Here's how the part is built. I have some questions about the finished solid (model axes, mm). Face numbers are marked on the shaded views. A direction names the side the tool comes from. Coordinates: 2 decimals unless noted, no trailing zeros. Write each loop counter-clockwise with the first axis right and the second up, starting at its lowest first coordinate (ties: lowest second). Pieces come first, ordered by that corner, then holes.
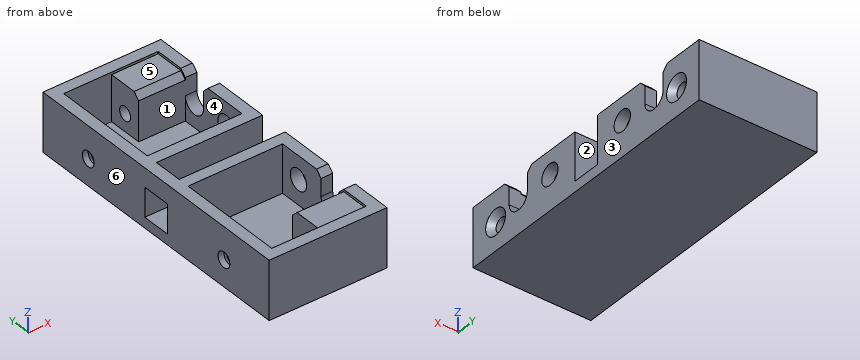
Autodesk Inventor part; units mm, degrees
ref_plane "YZ Plane" through (0, 0, 0) normal (1, 0, 0) x (0, 1, 0)
ref_plane "XZ Plane" through (0, 0, 0) normal (0, 1, 0) x (-1, 0, 0)
ref_plane "XY Plane" through (0, 0, 0) normal (0, 0, 1) x (1, 0, 0)
sketch "Sketch3" plane through (0, 0, 0) normal (0, 0, 1) x (1, 0, 0)
  line L0 (-10.1, 25) -> (10.1, 25)
  line L1 (10.1, 25) -> (10.1, -25)
  line L2 (10.1, -25) -> (-10.1, -25)
  line L3 (-10.1, -25) -> (-10.1, 25)
  point P0 (0, 0)
  dimension "d26" = 20.2
  dimension "d27" = 50
extrude "Extrusion3" add sketch "Sketch3" along normal blind 1.8
sketch "Sketch4" plane through (0, 0, 1.8) normal (0, 0, 1) x (1, 0, 0)
  line L0 (-8.1, 23) -> (8.1, 23)
  line L1 (8.1, -23) -> (-8.1, -23)
  line L2 (-8.1, 0) -> (-8.1, 2.5)
  line L3 (-8.1, 2.5) -> (8.1, 2.5)
  line L4 (8.1, 4.5) -> (-8.1, 4.5)
  line L5 (-8.1, 0) -> (-8.1, -2.5)
  line L6 (-8.1, -2.5) -> (8.1, -2.5)
  line L7 (8.1, -4.5) -> (-8.1, -4.5)
  line L8 (-8.1, 4.5) -> (-8.1, 23)
  line L9 (8.1, 23) -> (8.1, 4.5)
  line L10 (8.1, 2.5) -> (8.1, -2.5)
  line L11 (8.1, -4.5) -> (8.1, -23)
  line L12 (-10.1, 25) -> (-10.1, -25)
  line L13 (10.1, -25) -> (10.1, 25)
  line L14 (-10.1, 25) -> (10.1, 25)
  line L15 (10.1, 25) -> (10.1, -25)
  line L16 (10.1, -25) -> (-10.1, -25)
  line L17 (-10.1, -25) -> (-10.1, 25)
  line L18 (-8.1, -23) -> (-8.1, -4.5)
  line L19 (-8.1, -2.5) -> (-8.1, 2.5)
  point P0 (0, 0)
  dimension "d39" = 2.5
  dimension "d40" = 2.5
  dimension "d44" = 2
  dimension "d45" = 2
  dimension "d48" = 2
  dimension "d49" = 2
  dimension "d50" = 2
  dimension "d51" = 2
  dimension "d52" = 2
  dimension "d53" = 2
  dimension "d56" = 2
  dimension "d57" = 2
extrude "Extrusion4" add sketch "Sketch4" along normal blind 8.2
sketch "Sketch5" plane through (10.1, -25, 0) normal (1, 0, 0) x (0, 0, -1)
  line L0 (-1.8, 27.5) -> (-10, 27.5)
  line L1 (-1.8, 22.5) -> (-10, 22.5)
  line L2 (-10, 27.5) -> (-1.8, 27.5)
  line L3 (-1.8, 27.5) -> (-1.8, 22.5)
  line L4 (-1.8, 22.5) -> (-10, 22.5)
  line L5 (-10, 22.5) -> (-10, 27.5)
  point P0 (0, 25)
extrude "Extrusion5" cut sketch "Sketch5" against normal blind 8.2
sketch "Sketch6" plane through (-10.1, -25, 0) normal (-1, 0, 0) x (0, 0, 1)
  line L0 (1.8, 27.5) -> (1.8, 22.5)
  line L1 (1.8, 22.5) -> (6.8, 22.5)
  line L2 (6.8, 22.5) -> (6.8, 27.5)
  line L3 (6.8, 27.5) -> (1.8, 27.5)
  line L4 (1.8, 27.5) -> (1.8, 22.5)
  point P0 (0, 25)
  dimension "d60" = 5
  dimension "d61" = 5
extrude "Extrusion6" cut sketch "Sketch6" against normal blind 8.2
sketch "Sketch10" plane through (-10.1, -25, 0) normal (-1, 0, 0) x (0, 0, 1)
  line L0 (0, 0) -> (0, 50)
  line L1 (0, 0) -> (10, 0)
  point P0 (0, 25)
  point P1 (4.5, 10)
  point P2 (4.5, 40)
hole "Hole6" at (-10.1, -15, 4.5) at (-10.1, 15, 4.5) direction (1, 0, 0) diameter 2.6 depth 2 tip angle 118
sketch "Sketch11" plane through (0, 0, 1.8) normal (0, 0, 1) x (1, 0, 0)
  line L0 (8.1, -23) -> (8.1, -4.5)
  line L1 (8.1, -23) -> (0.1, -23)
  line L2 (0.1, -23) -> (0.1, -17)
  line L3 (0.1, -17) -> (8.1, -17)
  line L4 (8.1, -17) -> (8.1, -23)
  line L5 (10.1, 25) -> (10.1, -25)
  line L6 (8.1, 23) -> (0.1, 23)
  line L7 (0.1, 23) -> (0.1, 17)
  line L8 (0.1, 17) -> (8.1, 17)
  line L9 (8.1, 17) -> (8.1, 23)
  point P0 (0, 0)
  dimension "d143" = 8
  dimension "d144" = 6
extrude "Extrusion9" add sketch "Sketch11" along normal blind 7.8
sketch "Sketch12" plane through (10.1, -25, 0) normal (1, 0, 0) x (0, 0, -1)
  line L0 (0, 50) -> (0, 0)
  line L1 (0, 0) -> (-10, 0)
  circle A0 centre (-6, 10) radius 2
  line L2 (-1.8, 8) -> (-9.6, 8)
  line L3 (-10, 20.5) -> (-10, 2)
  line L4 (-6, 8) -> (-10, 8)
  line L5 (-10, 8) -> (-10, 12)
  line L6 (-10, 12) -> (-6, 12)
  line L7 (-6, 12) -> (-6, 8)
  line L8 (0, 25) -> (-4.8, 25)
  circle A1 centre (-6, 40) radius 2
  line L9 (-1.8, 42) -> (-9.6, 42)
  line L10 (-6, 42) -> (-10, 42)
  line L11 (-10, 42) -> (-10, 38)
  line L12 (-10, 38) -> (-6, 38)
  line L13 (-6, 38) -> (-6, 42)
  point P0 (-4.8, 5)
  point P1 (-6, 17)
  point P2 (-4.8, 45)
  point P3 (-6, 33)
  dimension "d153" = 4
hole "Hole7" at (10.1, -20, 4.8) at (10.1, 20, 4.8) direction (-1, 0, 0) diameter 2.4 depth 10 tip angle 118
hole "Hole8" at (10.1, -8, 6) at (10.1, 8, 6) direction (-1, 0, 0) diameter 3.6 depth 2 tip angle 118
extrude "Extrusion10" cut sketch "Sketch12" against normal blind 2
chamfer "Chamfer4" distance 1 angle 45 10 edges at (10.1, -20, 6) (-8.1, -15, 3.2) (10.1, 20, 6) (-8.1, 15, 3.2) (4.1, -17, 9.6) (4.1, 17, 9.6) (9.1, -17, 10) (9.1, 17, 10) (9.1, 13, 10) (9.1, -13, 10)
properties part number "digit_holder_A_no_hole"
1) Imagine slicing it at D-D on y = -8. Please give me the cut outline in (x, z).
Values follow:
outline: (-10.1, 0) - (10.1, 0) - (10.1, 4.2) - (8.1, 4.2) - (8.1, 1.8) - (-8.1, 1.8) - (-8.1, 10) - (-10.1, 10) - close; (8.1, 7.8) - (10.1, 7.8) - (10.1, 10) - (8.1, 10) - close
2) I need wall thicknesses on probe 1 along Y at (x, z) = (3, 4.8); probe 2 along Y at (x, z) = (-8, 7); probe 3 along Y at (x, z) = (4.75, 3.5). Which ranges of each line are inside material? Lowest first, please.
Values follow:
probe 1: y = -25 to -21.2, -18.8 to -17, -4.5 to -2.5, 2.5 to 4.5, 17 to 18.8, 21.2 to 25
probe 2: y = -25 to -23, -4.5 to -2.5, 2.5 to 4.5, 23 to 25
probe 3: y = -25 to -17, -4.5 to -2.5, 2.5 to 4.5, 17 to 25
3) Will these pins go through, and if not, where does the flat tip stop? pin 1 (2 mm diameter, centred on x = 8, y = -15, fed in from +Z); pin 2 (2.5 mm diameter, centred on x = 3.5, y = 20.5, fed in from +Z); pin 3 (2.5 mm diameter, centred on y = -15, z = 4.5, fed in from -X).
Values follow:
pin 1: stops at z = 4.27
pin 2: stops at z = 9.6
pin 3: stops at x = 8.1
4) On a 3-axis mill with a long thin cutter (end or side, diameter ignored), from which of +Z, -Z, +X, -X, +Y, -Y can I reach the whole of each face in a straight line? I mean the marked faces 5 and 6. Say none if no direction works.
Values follow:
face 5: +Z
face 6: +Z, -Z, -X, +Y, -Y
5) Imagine slicing it at C-C on x = 1.25. Please give me the cut outline in (y, z), then the cut area to 3 significant figures.
Values follow:
outline: (-25, 0) - (25, 0) - (25, 10) - (23, 10) - (23, 9.6) - (18, 9.6) - (17, 8.6) - (17, 1.8) - (4.5, 1.8) - (4.5, 10) - (2.5, 10) - (2.5, 1.8) - (-2.5, 1.8) - (-2.5, 10) - (-4.5, 10) - (-4.5, 1.8) - (-17, 1.8) - (-17, 8.6) - (-18, 9.6) - (-23, 9.6) - (-23, 10) - (-25, 10) - close; hole circle Ø2.4 at (-20, 4.8); hole circle Ø2.4 at (20, 4.8)
area: 239 mm2
6) Imagine slicing it at B-B on x = -3.5. Please give me the cut outline in (y, z), then the cut area to 3 significant figures.
Values follow:
outline: (-25, 0) - (25, 0) - (25, 10) - (23, 10) - (23, 1.8) - (4.5, 1.8) - (4.5, 10) - (2.5, 10) - (2.5, 1.8) - (-2.5, 1.8) - (-2.5, 10) - (-4.5, 10) - (-4.5, 1.8) - (-23, 1.8) - (-23, 10) - (-25, 10) - close
area: 156 mm2
7) We'd pull the mould along X, two halves only. Please class the marked faces 1, 2, 3 and 4: pulls with the +X half, pulls with the -X half, needs draft (parallel to the pull), parting line crosses it, or undercut.
Values follow:
face 1: undercut
face 2: needs draft
face 3: pulls with the +X half
face 4: undercut
8) Imagine slicing it at A-A on y = -2. Please give me the cut outline in (x, z).
Values follow:
outline: (-10.1, 0) - (10.1, 0) - (10.1, 1.8) - (-10.1, 1.8) - close; (-10.1, 6.8) - (-8.1, 6.8) - (-8.1, 10) - (-10.1, 10) - close
